For this review, use the dimensioned drawing (mm, ordinates from the lowest corner) and the shaded views. Give positions to 0.01 mm unless a question says otherwise; leave off trailing zeros. Loops run counter-clockwise (first coordinate to the right, second up) from the corner with the lowest first, then second, coordinate; pieces in that order, holes last. Notation, with made-up numbers: (5, -32.75) -> (15, -32.75) arc R23 ccw to (15, 5.25) -> close; hole circle Ø1 at (-25.5, -14). An arc over 180 degrees is marked (long way). Use a Markdown table: item, result. Add a question column.
1. For pin 1 Ø3 at (x, y) = (187.5, 3) entering from -Z; pin 2 Ø5 at (x, y) = (127.5, 3) entering from +Z (3 decimals); pin 3 Ø3 at (y, z) = (8, 101) entering from +X (3 decimals); pin 4 Ø5 at (y, z) = (4, 99.5) entering from -X (3 decimals), all flat-tipped, find the tip position at first contact; note any pin that passes through.
2. To check wall thickness, follow line 1 (X direction, y = 1.5, z = 49.5) (3 decimals); line 2 (Z direction, x = 61, y = 3) (3 decimals); line 3 (Z direction, x = 149.5, y = 5.25) (3 decimals). State the ranges of each line that lie inside material, in increasing order.
3. Add section A-A (z = 98). State the section outline as (x, y) points (3 decimals), and give its area (3 significant figures).
4. Add section B-B (y = 5.5). Count the separate pieces of the cut face and the enclosed holes in it, and give its area (3 significant figures).
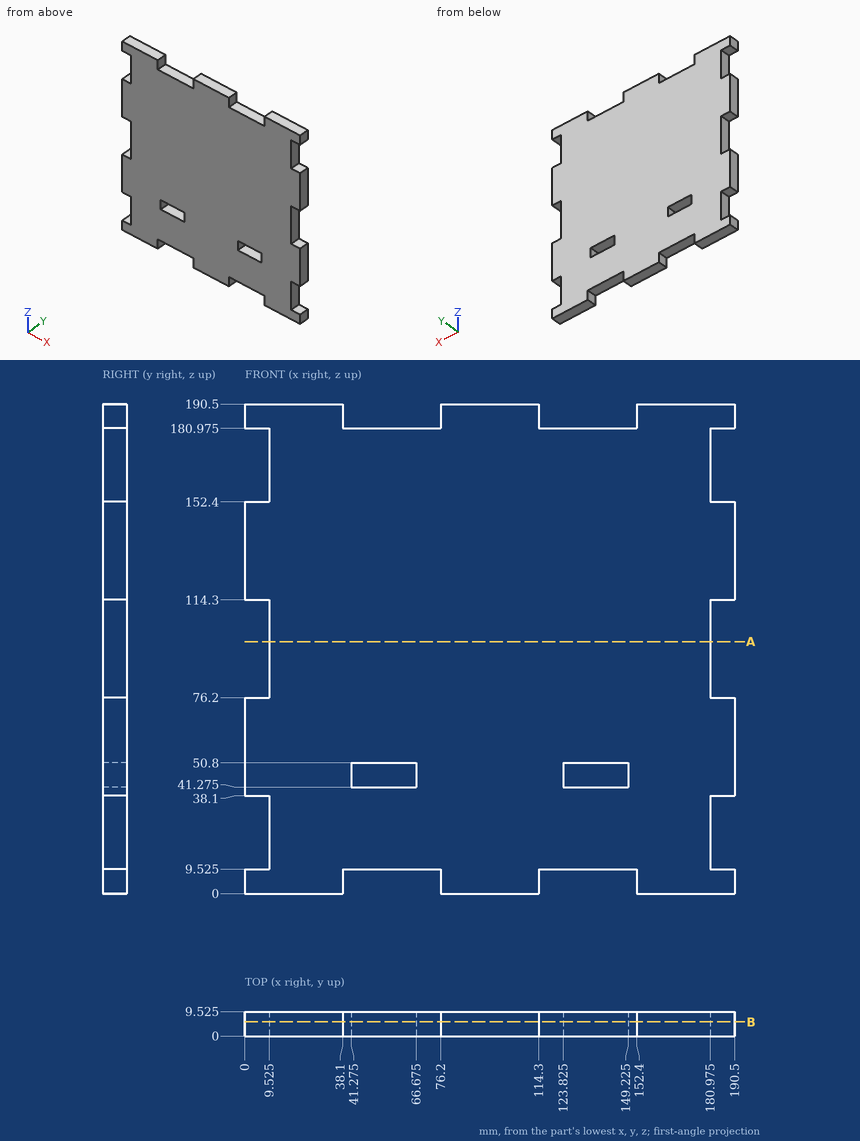
Taken from the geometry:
| question | item | result |
|---|---|---|
| 1 | pin 1 | stops at z = 0 |
| 1 | pin 2 | stops at z = 180.975 |
| 1 | pin 3 | stops at x = 180.975 |
| 1 | pin 4 | stops at x = 9.525 |
| 2 | line 1 | x = 0 to 41.275, 66.675 to 123.825, 149.225 to 190.5 |
| 2 | line 2 | z = 9.525 to 41.275, 50.8 to 180.975 |
| 2 | line 3 | z = 9.525 to 180.975 |
| 3 | outline | (9.525, 0) -> (180.975, 0) -> (180.975, 9.525) -> (9.525, 9.525) -> close |
| 3 | area | 1,630 mm^2 |
| 4 | separate pieces | 1 |
| 4 | enclosed holes | 2 |
| 4 | area | 32,500 mm^2 |
